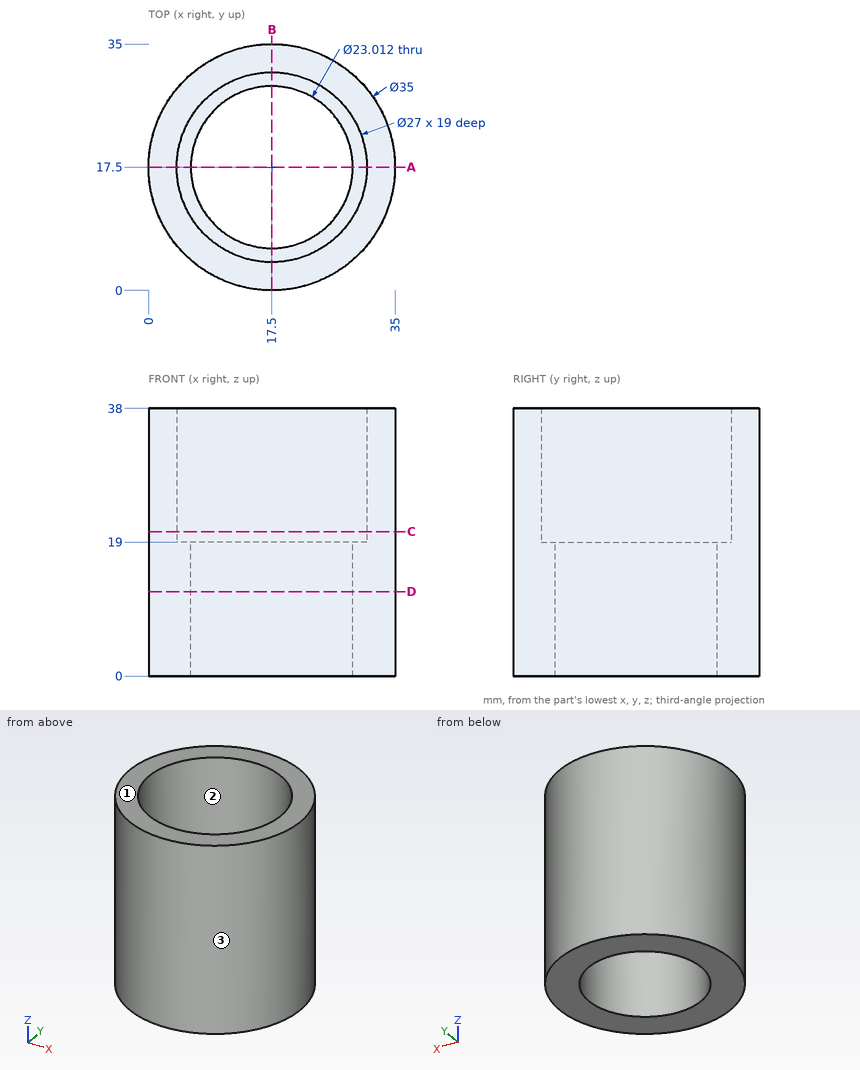
Geometry: see drawing. Coordinates: mm, zero at the bounding-box minimum. Round coordinates to 2 decimals unless told otherwise and drop trailing zeros. Loops run counter-clockwise (first coordinate to the right, second up) from the corner with the lowest first, then second, coordinate; pieces in that order, holes last. Notation, with made-up numbers: (-14, -1.5) - (35, -1.5) arc R32 ccw to (35, 30.5) - close; hole circle Ø6 at (27.5, -9). An arc over 180 degrees is marked (long way). One line per item, written item: value. Start each with the question number.
(1) Section D-D, the plane z = 12. Return loops of the section in (x, y).
(2) Section C-C, the plane z = 20.5. Return loops of the section in (x, y).
(3) Contact query for flat-ended pins moving along their axis: P1, Ø1.5, axis at x = 21.5, y = 5.5, coming from the +Z side; P2, Ø5, axis at x = 10, z = 19.5, coming from the -Y side; P3, Ø6, axis at y = 24.5, z = 20, coming from the -X side; P4, Ø8, axis at x = 13, y = 14.5, coming from the +Z side. Output: stop coordinate, or through.
(4) Draft query along X for the marked faces 1, 2 and 3. Return one class per face: +X half, -X half, draft (parallel to the pull), parting line (faces both ways), or undercut.
(5) Ray query, line 1 (Y direction, x = 17, z = 9) (1 decimal); line 2 (X direction, y = 17, z = 27); line 3 (Y direction, x = 17.5, z = 32.25). Return the intervals inside material, ascending. Write a range as [from, to].
(6) Section A-A, the plane y = 17.5. Return loops of the section in (x, z), plus the area to 3 significant figures.
Results below:
1. outline: circle Ø35 at (17.5, 17.5); hole circle Ø23.01 at (17.5, 17.5)
2. outline: circle Ø35 at (17.5, 17.5); hole circle Ø27 at (17.5, 17.5)
3. P1: z = 19
3. P2: y = 0.73
3. P3: x = 0.46
3. P4: through
4. face 1: draft
4. face 2: undercut
4. face 3: parting line
5. line 1: [0, 6], [29, 35]
5. line 2: [0.01, 4.01], [30.99, 34.99]
5. line 3: [0, 4], [31, 35]
6. outline: (0, 0) - (5.99, 0) - (5.99, 19) - (4, 19) - (4, 38) - (0, 38) - close; (29.01, 0) - (35, 0) - (35, 38) - (31, 38) - (31, 19) - (29.01, 19) - close
6. area: 380 mm^2
